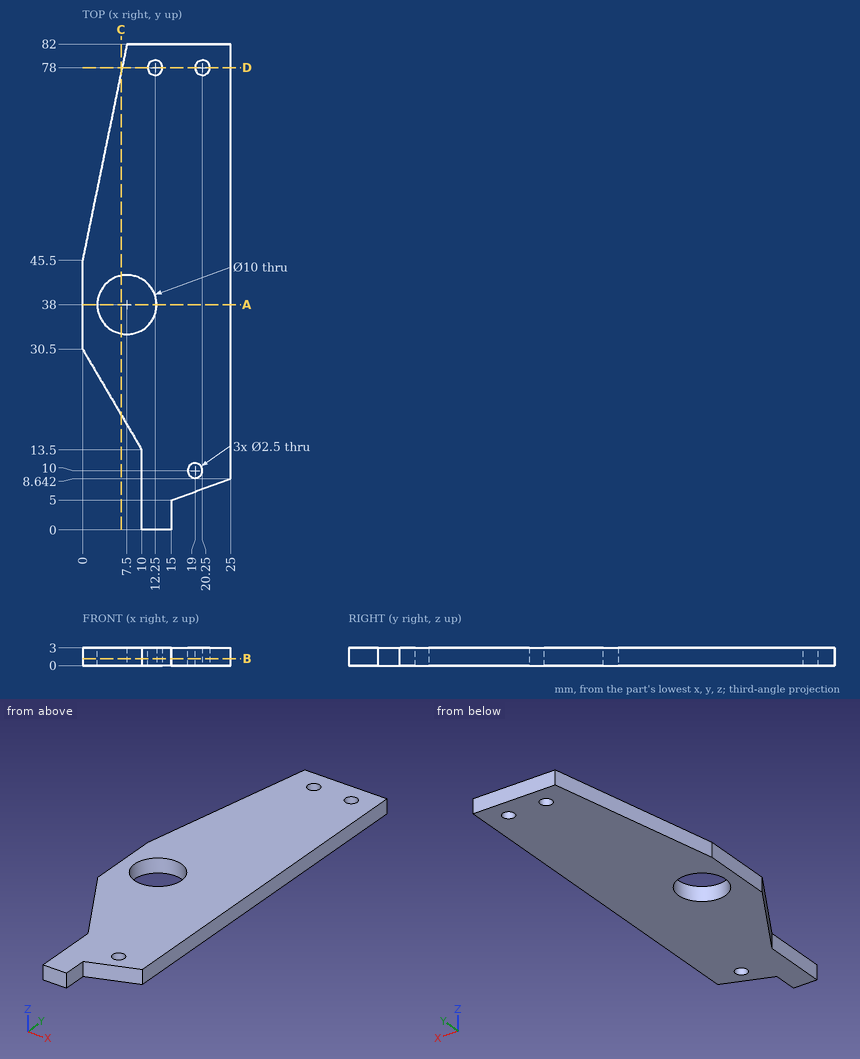
Input: dimensioned drawing with shaded views. Units: mm. Origin: part minimum x, y, z. Coordinates: 2 decimals unless noted, no trailing zeros. Write each loop counter-clockwise with the first axis right and the second up, starting at its lowest first coordinate (ties: lowest second). Pieces come first, ordered by that corner, then holes. Notation, with made-up numbers: M -19,-5 L 2,-5 A25 ccw 2,31 Z; hole C 14,22 d3. An arc over 180 degrees is marked long. Use one line per item in the form item = value.
Q1. Section B-B (z = 1.2). Return loops of the section in (x, y), plus the area to 3 significant figures.
Answer below:
outline = M 0,30.5 L 10,13.5 L 10,0 L 15,0 L 15,5 L 25,8.64 L 25,82 L 7.5,82 L 0,45.5 Z; hole C 7.5,38 d10; hole C 12.25,78 d2.5; hole C 19,10 d2.5; hole C 20.25,78 d2.5
area = 1,530 mm²
Q2. First-contact query: pin 1 (0.9 mm diameter, centred on y = 7, z = 1, fed in from -X); pin 2 (1.5 mm diameter, centred on y = 19.5, z = 2.5, fed in from -X). Flat tips, straight axial feed; report the tip coordinate or a pass-through.
Answer below:
pin_1 = 10
pin_2 = 6.03
Q3. Material intervals for probe 1 along X at (y, z) = (67, 1.15); probe 2 along Y at (x, z) = (21, 0.9) (1 decimal); probe 3 along X at (y, z) = (10.5, 1.55) (1 decimal), sorted ascending. Write a range as from..to.
Answer below:
probe_1 = 4.42..25
probe_2 = 7.2..77, 79..82
probe_3 = 10..17.9, 20.1..25
Q4. Section D-D (y = 78). Return loops of the section in (x, z).
Answer below:
outline = M 6.68,0 L 11,0 L 11,3 L 6.68,3 Z; M 13.5,0 L 19,0 L 19,3 L 13.5,3 Z; M 21.5,0 L 25,0 L 25,3 L 21.5,3 Z
Q5. Section C-C (x = 6.5). Return loops of the section in (y, z).
Answer below:
outline = M 19.45,0 L 33.1,0 L 33.1,3 L 19.45,3 Z; M 42.9,0 L 77.13,0 L 77.13,3 L 42.9,3 Z
Q6. Section A-A (y = 38). Return loops of the section in (x, z).
Answer below:
outline = M 0,0 L 2.5,0 L 2.5,3 L 0,3 Z; M 12.5,0 L 25,0 L 25,3 L 12.5,3 Z
